Study the drawing (mm; zero at the part's minimum x, y, z) and answer. A direction names the side the tool comes from. Give positions to 0.01 mm unless a question says otherwise; leave off trailing zeros. Write each loop counter-clockwise with the first axis right and the second up, starting at its lowest first coordinate (ties: lowest second). Pieces come first, ordered by that corner, then holes. Notation, with made-up numbers: (43.5, 49) - (92.5, 49) arc R32 ccw to (92.5, 85) - close; hole circle Ø11 at (54.5, 59.25). An arc over 180 degrees is marked (long way). Return JSON: item names as keys, results as strings.
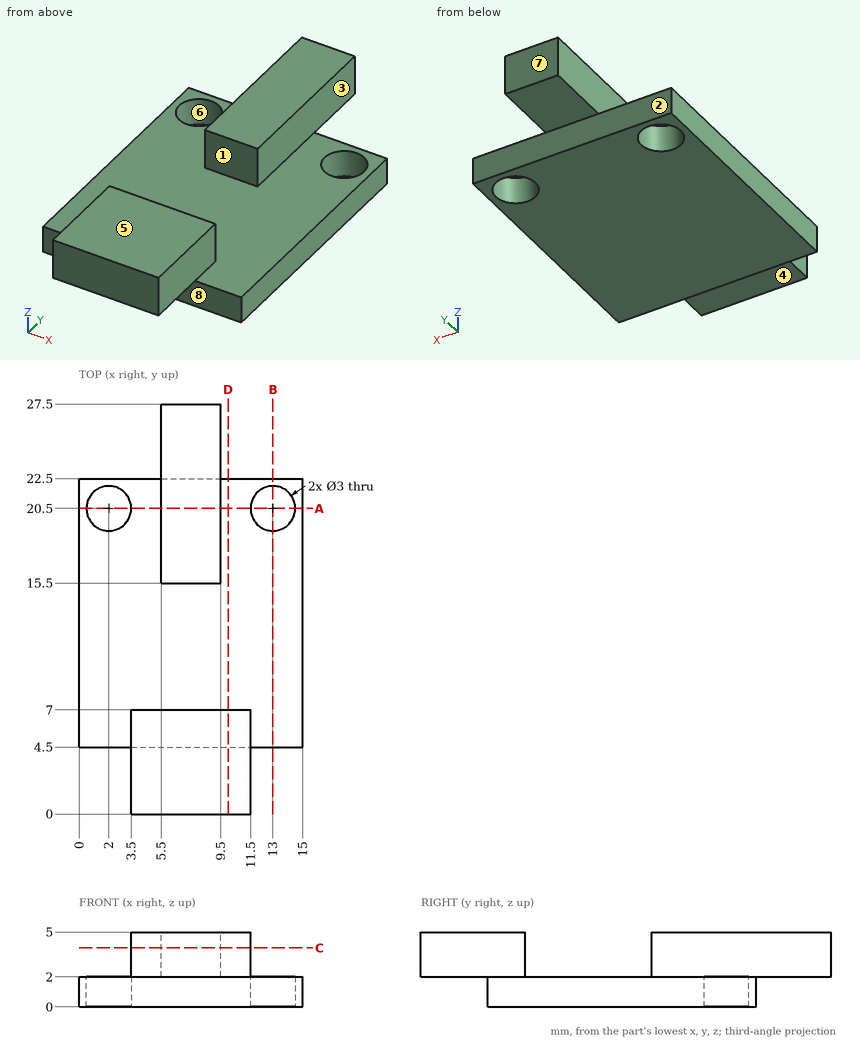
Item 1: Flat-ended cylindrical pins translate along their axes: P1, Ø1.5, axis at y = 18.5, z = 3, coming from the -X side; P2, Ø1.3, axis at x = 6, y = 1.5, coming from the -Z side; P3, Ø2.5, axis at x = 2, y = 20.5, coming from the +Z side; P4, Ø0.6, axis at x = 10, z = 1, coming from the -Y side. Find the tip coordinate at first contact, or state that the pin passes through.
Answer below:
{"P1": "stops at x = 5.5", "P2": "stops at z = 2", "P3": "passes through", "P4": "stops at y = 4.5"}
Item 2: A cutting plane is placed at D-D on x = 10. Determine the outline of the cut face in (y, z), then the cut area to 3 significant figures.
Answer below:
{"outline": "(0, 2) - (4.5, 2) - (4.5, 0) - (22.5, 0) - (22.5, 2) - (7, 2) - (7, 5) - (0, 5) - close", "area": "57.0 mm²"}
Item 3: A cutting plane is placed at C-C on z = 3.95. Determine the outline of the cut face in (x, y), then the cut area to 3 significant figures.
Answer below:
{"outline": "(3.5, 0) - (11.5, 0) - (11.5, 7) - (3.5, 7) - close; (5.5, 15.5) - (9.5, 15.5) - (9.5, 27.5) - (5.5, 27.5) - close", "area": "104 mm²"}
Item 4: A cutting plane is placed at B-B on x = 13. Determine the outline of the cut face in (y, z).
Answer below:
{"outline": "(4.5, 0) - (19, 0) - (19, 2) - (4.5, 2) - close; (22, 0) - (22.5, 0) - (22.5, 2) - (22, 2) - close"}
Item 5: A cutting plane is placed at A-A on y = 20.5. Determine the outline of the cut face in (x, z).
Answer below:
{"outline": "(0, 0) - (0.5, 0) - (0.5, 2) - (0, 2) - close; (3.5, 0) - (11.5, 0) - (11.5, 2) - (9.5, 2) - (9.5, 5) - (5.5, 5) - (5.5, 2) - (3.5, 2) - close; (14.5, 0) - (15, 0) - (15, 2) - (14.5, 2) - close"}
Item 6: For the marked faces 1, 2, 3 and 4, determine the directions among +Z, -Z, +X, -X, +Y, -Y from which every point of the face is accessible in a straight line to the end or side of a thin tool.
Answer below:
{"face 1": "+Z, +X, -X", "face 2": "-Z, +X, -X, +Y", "face 3": "+Z, +X, +Y", "face 4": "-Z, +X, -X, -Y"}
Item 7: The mould has two halves that part along Y. Classify the marked faces 5, 6, 7 and 8: +Y half, -Y half, draft (parallel to the pull), parting line (faces both ways), or undercut.
Answer below:
{"face 5": "draft", "face 6": "undercut", "face 7": "+Y half", "face 8": "-Y half"}
Item 8: Consider L1, parallel to Y at x = 2, z = 1.3; L2, parallel to X at y = 25.25, z = 4.5; L3, parallel to Z at x = 2, y = 9. Determine where each line is inside the solid, lowest interval first.
Answer below:
{"L1": "y = 4.5 to 19, 22 to 22.5", "L2": "x = 5.5 to 9.5", "L3": "z = 0 to 2"}
